Geometry: final body of the model. Coordinates: model frame, mm. Face numbers are marked on the shaded views. Give positions to 0.01 mm unless a question says otherwise; leave off trailing zeros. Write each loop counter-clockwise with the first axis right and the second up, starting at its lowest first coordinate (ties: lowest second). Pieces come first, ordered by that corner, then holes.
Q1. Section C-C (y = 1.3). State how many separate pieces and enclosed holes the cut face has, plus the area to 3 significant figures.
Q2. Mould query, pull axis Z, two halves, no side actions, for the marked faces 1, 2 and 3. Classes: +Z half, -Z half, draft (parallel to the pull), parting line (faces both ways), or undercut.
Q3. Section D-D (z = -63.5). Return the cut outline in (x, y).
Q4. Pin query (flat end, axial travel): pin 1 Ø6 at (x, z) = (14, -53.5) entering from +Y; pin 2 Ø0.6 at (y, z) = (1.5, -120.5) entering from -X; pin 3 Ø0.6 at (x, y) = (14, 1) entering from +Z. Return the tip coordinate at first contact, or that it passes through.
Q5. Line query: line 1 (Z direction, x = 18, y = 1.35); line 2 (Z direction, x = 5.25, y = 0.2); line 3 (Y direction, x = 16.5, z = -67.5). Output: solid intervals per line, ascending.
Q6. Section B-B (z = -32.5). Return the cut outline in (x, y), plus the area to 3 significant figures.
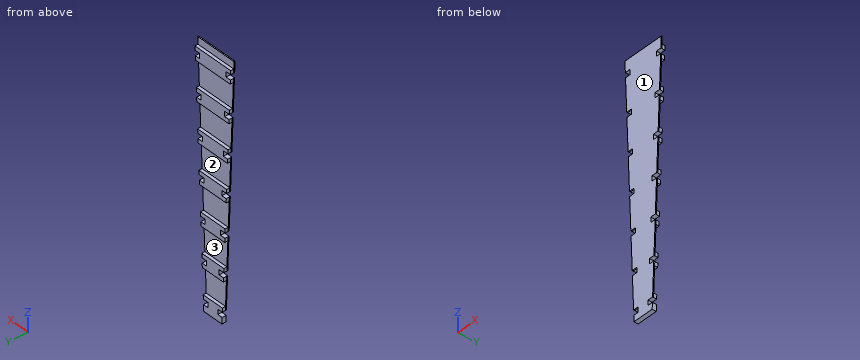
from build123d import *

# Parameters (mm, degrees)
BOSS_EXTRUDE1_DEPTH = 0.5
BOSS_EXTRUDE2_DEPTH = 1.5


with BuildPart() as part:
    # Sketch2 → Boss-Extrude1 (new body)
    with BuildSketch(Plane(origin=(0, 0, 0), x_dir=(1, 0, 0), z_dir=(0, 1, 0))):
        Polygon((0.219191575, 5.479789367), (0, 0), (20, 0), (19.780808425, 5.479789367), (17.280808425, 5.479789367), (17.280808425, 7.979789367), (19.680808425, 7.979789367), (19.021415697, 24.464607583), (16.521415698, 24.464607583), (16.521415698, 26.964607583), (18.921415697, 26.964607583), (18.262022968, 43.449425798), (15.76202297, 43.449425798), (15.76202297, 45.949425798), (18.162022968, 45.949425798), (17.502630239, 62.434244014), (15.002630242, 62.434244014), (15.002630242, 64.934244014), (17.402630239, 64.934244014), (16.743237511, 81.41906223), (14.243237514, 81.41906223), (14.243237514, 83.91906223), (16.643237511, 83.91906223), (15.983844782, 100.403880446), (13.483844787, 100.403880446), (13.483844787, 102.903880446), (15.883844782, 102.903880446), (15.224452054, 119.388698661), (12.724452059, 119.388698661), (12.724452059, 121.888698661), (15.124452054, 121.888698661), (15, 125), (5, 125), (4.875547946, 121.888698661), (7.275547941, 121.888698661), (7.275547941, 119.388698661), (4.775547941, 119.388698661), (4.116155218, 102.903880446), (6.516155213, 102.903880446), (6.516155213, 100.403880446), (4.016155213, 100.403880446), (3.356762489, 83.91906223), (5.756762486, 83.91906223), (5.756762486, 81.41906223), (3.256762486, 81.41906223), (2.597369761, 64.934244014), (4.997369758, 64.934244014), (4.997369758, 62.434244014), (2.497369758, 62.434244014), (1.837977032, 45.949425798), (4.23797703, 45.949425798), (4.23797703, 43.449425798), (1.73797703, 43.449425798), (1.078584303, 26.964607583), (3.478584302, 26.964607583), (3.478584302, 24.464607583), (0.978584302, 24.464607583), (0.319191575, 7.979789367), (2.719191575, 7.979789367), (2.719191575, 5.479789367), align=None)
    extrude(amount=BOSS_EXTRUDE1_DEPTH)

    # Sketch3 → Boss-Extrude2 (add)
    with BuildSketch(Plane(origin=(0, 0.5, 0), x_dir=(1, 0, 0), z_dir=(0, 1, 0))):
        Polygon((0.219191575, 5.479789367), (0.14, 3.5), (19.86, 3.5), (19.780808425, 5.479789367), (17.280808425, 5.479789367), (17.280808425, 7.979789367), (19.680808425, 7.979789367), (19.6, 10), (0.4, 10), (0.319191575, 7.979789367), (2.719191575, 7.979789367), (2.719191575, 5.479789367), align=None)
        Polygon((0.978584302, 24.464607561), (0.898584302, 22.464607561), (19.101415698, 22.464607561), (19.021415697, 24.464607583), (16.521415698, 24.464607583), (16.521415698, 26.964607583), (18.921415697, 26.964607583), (18.841415697, 28.964607583), (1.158584303, 28.964607583), (1.078584303, 26.964607583), (3.478584302, 26.964607583), (3.478584302, 24.464607583), align=None)
        Polygon((1.73797703, 43.449425755), (1.657977032, 41.449425798), (18.342022968, 41.449425798), (18.262022968, 43.449425798), (15.76202297, 43.449425798), (15.76202297, 45.949425798), (18.162022968, 45.949425798), (18.082022968, 47.949425798), (1.917977032, 47.949425798), (1.837977032, 45.949425798), (4.23797703, 45.949425798), (4.23797703, 43.449425798), align=None)
        Polygon((2.497369758, 62.434243949), (2.417369761, 60.434244014), (17.582630239, 60.434244014), (17.502630239, 62.434244014), (15.002630242, 62.434244014), (15.002630242, 64.934244014), (17.402630239, 64.934244014), (17.322630239, 66.934244014), (2.677369761, 66.934244014), (2.597369761, 64.934244014), (4.997369758, 64.934244014), (4.997369758, 62.434244014), align=None)
        Polygon((3.256762486, 81.419062142), (3.176762489, 79.41906223), (16.823237511, 79.41906223), (16.743237511, 81.41906223), (14.243237514, 81.41906223), (14.243237514, 83.91906223), (16.643237511, 83.91906223), (16.563237511, 85.91906223), (3.436762489, 85.91906223), (3.356762489, 83.91906223), (5.756762486, 83.91906223), (5.756762486, 81.41906223), align=None)
        Polygon((4.016155213, 100.403880336), (3.936155218, 98.403880446), (16.063844782, 98.403880446), (15.983844782, 100.403880446), (13.483844787, 100.403880446), (13.483844787, 102.903880446), (15.883844782, 102.903880446), (15.803844782, 104.903880446), (4.196155218, 104.903880446), (4.116155218, 102.903880446), (6.516155213, 102.903880446), (6.516155213, 100.403880446), align=None)
        Polygon((4.775547941, 119.38869853), (4.695547946, 117.388698661), (15.304452054, 117.388698661), (15.224452054, 119.388698661), (12.724452059, 119.388698661), (12.724452059, 121.888698661), (15.124452054, 121.888698661), (15, 125), (5, 125), (4.875547946, 121.888698661), (7.275547941, 121.888698661), (7.275547941, 119.388698661), align=None)
    extrude(amount=BOSS_EXTRUDE2_DEPTH)


solid = part.part
Computed:
1. separate pieces: 7
1. enclosed holes: 0
1. area: 604 mm2
2. face 1: draft
2. face 2: undercut
2. face 3: undercut
3. outline: (5, 0) - (15, 0) - (15, 2) - (5, 2) - close
4. pin 1: stops at y = 0.5
4. pin 2: stops at x = 7.28
4. pin 3: stops at z = -3.5
5. line 1: z = -47.95 to -45.95, -43.45 to -41.45, -28.96 to -26.96, -24.46 to -22.46, -10 to -7.98, -5.48 to -3.5
5. line 2: z = -125 to -121.89, -119.39 to -102.9, -100.4 to -83.92, -81.42 to 0
5. line 3: y = 0 to 0.5
6. outline: (1.3, 0) - (18.7, 0) - (18.7, 0.5) - (1.3, 0.5) - close
6. area: 8.70 mm2
